Build history of the part. All positions in model axes, mm. A direction names the side the tool comes from. Coordinates: 2 decimals unless noted, no trailing zeros. Write each loop counter-clockwise with the first axis right and the second up, starting at its lowest first coordinate (ties: lowest second). Pieces come first, ordered by that corner, then holes.
```python
from build123d import *

# Parameters (mm, degrees)
SKETCH_R      = 2.75
SKETCH_R_2    = 1.25
PAD_DEPTH     = 2
SKETCH001_R   = 4.75
SKETCH001_R_2 = 2.75
PAD001_DEPTH  = 2
SKETCH002_R   = 2.75
PAD002_DEPTH  = 2.5
SKETCH003_R   = 2.75
SKETCH003_R_2 = 1.25
PAD003_DEPTH  = 2
POCKET_DEPTH  = 1


with BuildPart() as part:
    # Sketch → Pad (new body)
    with BuildSketch(Plane.XY):
        with BuildLine():
            ThreePointArc((6.964912, -0.7), (0, 7), (-6.964912, -0.7))
            Line((-6.964912, -0.7), (-4.974937, -20.5))
            ThreePointArc((-4.974937, -20.5), (0, -25), (4.974937, -20.5))
            Line((6.964912, -0.7), (4.974937, -20.5))
        make_face()
        Circle(SKETCH_R, mode=Mode.SUBTRACT)
        with Locations((0, -20)):
            Circle(SKETCH_R_2, mode=Mode.SUBTRACT)
    extrude(amount=PAD_DEPTH)

    # Sketch001 (on DatumPlane) → Pad001 (join)
    with BuildSketch(Plane.XY.offset(2)):
        Circle(SKETCH001_R)
        Circle(SKETCH001_R_2, mode=Mode.SUBTRACT)
    extrude(amount=PAD001_DEPTH)

    # Sketch002 (on DatumPlane) → Pad002 (join)
    with BuildSketch(Plane.XY.offset(2)):
        with BuildLine():
            Line((-5.950745, -10.790833), (5.298025, -17.285314))
            Line((6.964912, -0.7), (5.298025, -17.285314))
            ThreePointArc((6.964912, -0.7), (0, 7), (-6.964912, -0.7))
            Line((-6.964912, -0.7), (-5.950745, -10.790833))
        make_face()
        Circle(SKETCH002_R, mode=Mode.SUBTRACT)
    extrude(amount=PAD002_DEPTH)

    # Sketch003 (on DatumPlane) → Pad003 (join)
    with BuildSketch(Plane.XY.offset(4.5)):
        with BuildLine():
            ThreePointArc((6.964912, -0.7), (0, 7), (-6.964912, -0.7))
            Line((-6.964912, -0.7), (-4.974937, -20.5))
            ThreePointArc((-4.974937, -20.5), (0, -25), (4.974937, -20.5))
            Line((6.964912, -0.7), (4.974937, -20.5))
        make_face()
        Circle(SKETCH003_R, mode=Mode.SUBTRACT)
        with Locations((0, -20)):
            Circle(SKETCH003_R_2, mode=Mode.SUBTRACT)
    extrude(amount=PAD003_DEPTH)

    # Sketch007 (on DatumPlane) → Pocket (cut)
    with BuildSketch(Plane.XY.offset(6.5)):
        Polygon((2.2, -21.270171), (2.2, -18.729829), (0, -17.459659), (-2.2, -18.729829), (-2.2, -21.270171), (0, -22.540341), align=None)
    extrude(amount=-POCKET_DEPTH, mode=Mode.SUBTRACT)

    # Sketch008 → Groove (revolve, cut)
    with BuildSketch(Plane.YZ):
        Polygon((-20, 0), (-18.1, 0), (-18.9, 1), (-20, 1), align=None)
    revolve(axis=Axis((0, -20, 0), (0, 0, 1)), mode=Mode.SUBTRACT)


solid = part.part
```
1. Probe line 1 along Y through (x, z) = (0, 4.8); line 2 along Y through (x, z) = (-1, 6.25); line 3 along Y through (x, z) = (1, 3.25). List the from-to ranges inside material, lowest first.
Computed values:
line 1: y = -25 to -21.25, -18.75 to -2.75, 2.75 to 7
line 2: y = -24.9 to -21.96, -18.04 to -2.56, 2.56 to 6.93
line 3: y = -14.8 to -2.56, 2.56 to 6.93
2. Saw through at D-D on z = 1.5. List the corners of the cut face in (x, y), plus the area to 3 significant figures.
Computed values:
outline: (-6.96, -0.7) - (-4.97, -20.5) arc R5 ccw to (4.97, -20.5) - (6.96, -0.7) arc R7 ccw (long way) to start; hole circle Ø5.5 at (0, 0); hole circle Ø2.5 at (0, -20)
area: 329 mm2
3. Saw through at C-C on y = -20. List the corners of the cut face in (x, z), plus the area to 3 significant figures.
Computed values:
outline: (-5.03, 0) - (-1.9, 0) - (-1.25, 0.81) - (-1.25, 2) - (-5.03, 2) - close; (-5.03, 4.5) - (-1.25, 4.5) - (-1.25, 5.5) - (-2.2, 5.5) - (-2.2, 6.5) - (-5.03, 6.5) - close; (1.25, 0.81) - (1.9, 0) - (5.03, 0) - (5.03, 2) - (1.25, 2) - close; (1.25, 4.5) - (5.03, 4.5) - (5.03, 6.5) - (2.2, 6.5) - (2.2, 5.5) - (1.25, 5.5) - close
area: 27.8 mm2
4. Flat gauge pins, fed straight in: pin 1 (0.5 mm diameter, centred on y = -20.5, z = 6, fed in from +X); pin 2 (4 mm diameter, centred on x = 0, y = -20, fed in from +Z); pin 3 (2 mm diameter, centred on y = -4.5, z = 4, fed in from +X); pin 4 (3.5 mm diameter, centred on x = 0, y = 0, fed in from +Z). Where does each tip first touch, or does it go through?
Computed values:
pin 1: stops at x = 5
pin 2: stops at z = 5.5
pin 3: stops at x = 6.68
pin 4: passes through
5. Mould opens along X. For faces 1 (the face through (-0.596, -2.685, 3.204)), 2 (the face through (0, -9, 6.5)), 3 (the face through (0, 7, 3)) say: +X half, -X half, draft (parallel to the pull), parting line (faces both ways), or undercut.
Computed values:
face 1: undercut
face 2: draft
face 3: parting line
6. Saw through at B-B on z = 3.75. List the corners of the cut face in (x, y), plus the area to 3 significant figures.
Computed values:
outline: (-6.96, -0.7) - (-5.95, -10.79) - (5.3, -17.29) - (6.96, -0.7) arc R7 ccw (long way) to start; hole circle Ø5.5 at (0, 0)
area: 232 mm2
7. Saw through at A-A on y = 0. List the corners of the cut face in (x, z), plus the area to 4 significant figures.
Computed values:
outline: (-7, 0) - (-2.75, 0) - (-2.75, 6.5) - (-7, 6.5) - close; (2.75, 0) - (7, 0) - (7, 6.5) - (2.75, 6.5) - close
area: 55.25 mm2
8. 3-axis set-ups, long thin cutter, end or side, ignore diameter. For faces 4 (the face through (-0.27, -21.22, 4.99)), 5 (the face through (0, -18, 2)), 6 (the face through (-1.085, -18.086, 6.007)): which of +Z, -Z, +X, -X, +Y, -Y reach the whole face in a straight line?
Computed values:
face 4: +Z, -Z
face 5: -X, -Y
face 6: +Z
